For this review, take the finished solid that the model builds, in its own axes (mm). A direction names the side the tool comes from. Give positions to 0.01 mm unless a question says otherwise; leave off trailing zeros. Write each loop counter-clockwise with the first axis right and the second up, starting at its lowest first coordinate (ties: lowest second). Pieces come first, ordered by that corner, then holes. Notation, with made-up numbers: (49.25, -8.5) -> (64.25, -8.5) arc R6 ccw to (64.25, 0.5) -> close; hole circle Ø5 at (-11.75, 7.5). An arc over 180 degrees is marked (long way). Answer as CSV lines item,"result".
Autodesk Inventor part; units mm, degrees
ref_plane "YZ Plane" through (0, 0, 0) normal (1, 0, 0) x (0, 1, 0)
ref_plane "XZ Plane" through (0, 0, 0) normal (0, 1, 0) x (-1, 0, 0)
ref_plane "XY Plane" through (0, 0, 0) normal (0, 0, 1) x (1, 0, 0)
sketch "Sketch1" plane through (0, 0, 0) normal (0, 0, 1) x (1, 0, 0)
  line L0 (0, 3) -> (0, -3)
  line L1 (0, -3) -> (0.75, -3)
  line L2 (0.75, -3) -> (1, -2.75)
  line L3 (1, -2.75) -> (1, 0.9)
  line L4 (1.1, 1) -> (1.65, 1)
  line L5 (1.9, 1.25) -> (1.9, 2.75)
  line L6 (1.65, 3) -> (0, 3)
  arc A0 (1.1, 1) -> (1, 0.9) centre (1.1, 0.9) ccw
  line L7 (1.65, 3) -> (1.9, 2.75)
  line L8 (1.65, 1) -> (1.9, 1.25)
  point P0 (0, 0)
  point P1 (1.9, 1)
  point P2 (1.9, 3)
  point P3 (0, 0)
  dimension "d0" = 3.8
  dimension "d1" = 2
  dimension "d3" = 2
  dimension "d4" = 2.2
  dimension "d5" = 135
  dimension "d6" = 0.25
  dimension "d7" = 4
  dimension "d18" = 0.25
revolve "Revolution1" add sketch "Sketch1" angle 360 about axis through (0, 3, 0) along (0, -1, 0)
sketch "Sketch2" plane through (0, 3, 0) normal (0, 1, 0) x (1, 0, 0)
  line L0 (0, -0.866) -> (-0.75, -0.433)
  line L1 (-0.75, -0.433) -> (-0.75, 0.433)
  line L2 (-0.75, 0.433) -> (0, 0.866)
  line L3 (0, 0.866) -> (0.75, 0.433)
  line L4 (0.75, 0.433) -> (0.75, -0.433)
  line L5 (0.75, -0.433) -> (0, -0.866)
  point P0 (0, 0)
  point P1 (0, 0)
  dimension "d11" = 1.5
extrude "Extrusion1" cut sketch "Sketch2" against normal blind 1.5
thread "Thread1"
sketch "Sketch3" plane through (0, 0, 0) normal (1, 0, 0) x (0, 1, 0)
  line L0 (3, 0.866) -> (3, 0.433)
  line L1 (3, 0.866) -> (2.5, 0.366)
  line L2 (2.5, 0.366) -> (3, 0.366)
  line L3 (3, 0.366) -> (3, 0.866)
  line L4 (-0.6, 0) -> (3.6, 0)
  point P0 (0, 0)
  dimension "d16" = 0.5
revolve "Revolution2" cut sketch "Sketch3" angle 360 about axis through (0, -10, 0) along (0, 1, 0)
properties part number "Bolt_M2x0.4_4mm_SH" material "Stainless Steel"
Q1. Add section C-C (y = -0.5). Write out the cut boundary in (x, z), plus the area to 3 significant figures.
Answer block:
outline,"circle Ø2 at (0, 0)"
area,"3.14 mm2"
Q2. Add section B-B (z = 0). Write out the cut boundary in (x, y).
Answer block:
outline,"(-1.9, 1.25) -> (-1.65, 1) -> (-1.1, 1) arc R0.1 cw to (-1, 0.9) -> (-1, -2.75) -> (-0.75, -3) -> (0.75, -3) -> (1, -2.75) -> (1, 0.9) arc R0.1 cw to (1.1, 1) -> (1.65, 1) -> (1.9, 1.25) -> (1.9, 2.75) -> (1.65, 3) -> (0.87, 3) -> (0.75, 2.88) -> (0.75, 1.5) -> (-0.75, 1.5) -> (-0.75, 2.88) -> (-0.87, 3) -> (-1.65, 3) -> (-1.9, 2.75) -> close"
Q3. Draft analysis for pull direction X (two halves, no side actions). For faces 3 (the cylindrical face through (0, -1, 1)), 4 (the flat face through (0.75, 2, 0)), 5 (the flat face through (0, -3, 0)), state which applies: released by +X, released by -X, zero draft, split by the parting line, or undercut.
Answer block:
face 3,"split by the parting line"
face 4,"undercut"
face 5,"zero draft"
Q4. Add section A-A (y = 2). Write out the cut boundary in (x, z).
Answer block:
outline,"circle Ø3.8 at (0, 0); hole (-0.75, -0.43) -> (0, -0.87) -> (0.75, -0.43) -> (0.75, 0.43) -> (0, 0.87) -> (-0.75, 0.43) -> close"
Q5. For faces 1 (the flat face through (-0.75, 2, 0)), 2 (the cylindrical face through (-1.9, 2.01, -0.08)), list the 3-axis set-ups (+Z, -Z, +X, -X, +Y, -Y) from which the entire face can be reached by the end or side of a thin tool; tool diameter is ignored.
Answer block:
face 1,"+Y"
face 2,"+Y, -Y"
Q6. To check wall thickness, follow probe 1 along Y at (x, z) = (-1.2, -0.4); probe 2 along Y at (x, z) = (0.15, 0.4); probe 3 along X at (y, z) = (-0.5, 0.2). State the ranges of each line that lie inside material, in increasing order. Write a range as [from, to].
Answer block:
probe 1,"y = [1, 3]"
probe 2,"y = [-3, 1.5]"
probe 3,"x = [-0.98, 0.98]"
